The listing builds one solid part. Answer for the finished solid, in the listing's coordinates (mm). Give positions to 0.01 mm unless a question says otherwise; leave off trailing zeros. Write each loop counter-clockwise with the first axis right and the second up, starting at its lowest first coordinate (ties: lowest second). Pieces come first, ordered by that corner, then holes. Notation, with made-up numbers: (-31, 60) -> (2, 60) arc R9 cw to (2, 71) -> close; hole circle Ø5 at (81.5, 73). An arc over 180 degrees is marked (long way). One line per question, with ' | ' between items.
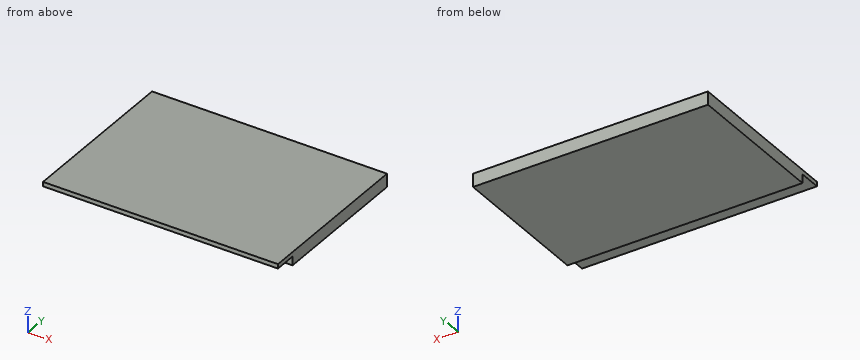
from build123d import *

# Parameters (mm, degrees)
F0_W     = 127
F0_H     = 79.375
F1_DEPTH = 7.5
F0_W_2   = 3.175
F0_H_2   = 12.7
F2_DEPTH = 2.5


with BuildPart() as f1:
    # F0 (on Top) → F1 (new body)
    with BuildSketch(Plane.XY):
        Polygon((85.0653162807, 76.807467067), (-48.2846837193, 76.807467067), (-48.2846837193, -5.742532933), (-45.1096837193, -5.742532933), (-45.1096837193, 73.632467067), (81.8903162807, 73.632467067), (81.8903162807, -5.742532933), (85.0653162807, -5.742532933), align=None)
        with Locations((18.3903162807, 33.944967067)):
            Rectangle(F0_W, F0_H)
    extrude(amount=-F1_DEPTH)

    # F0 (on Top) → F2 (join)
    with BuildSketch(Plane.XY):
        with Locations((-46.6971837193, -12.092532933)):
            Rectangle(F0_W_2, F0_H_2)
        with Locations((83.4778162807, -12.092532933)):
            Rectangle(F0_W_2, F0_H_2)
        with Locations((18.3903162807, -12.092532933)):
            Rectangle(F0_W, F0_H_2)
    extrude(amount=-F2_DEPTH)


solid = f1.part
Item 1: A flat-ended cylindrical pin translates along its axis: pin 1 (6 mm diameter, centred on x = 32, y = 15.5, fed in from +Z). Find the tip coordinate at first contact, or state that the pin passes through.
Answers below:
pin 1: z = 0
Item 2: Find section B-B (z = -6.25). Write down the section's boundary in (x, y), then the cut area to 3 significant figures.
Answers below:
outline: (-48.28, -5.74) -> (85.07, -5.74) -> (85.07, 76.81) -> (-48.28, 76.81) -> close | area: 11,000 mm²
Item 3: Consider line 1 (Y direction, x = 5.5, z = -6.25); line 2 (Z direction, x = -34, y = -9). Determine where each line is inside the solid, lowest interval first. Write a range as [from, to].
Answers below:
line 1: [-5.74, 76.81] | line 2: [-2.5, 0]
Item 4: Find section A-A (x = 47.5). Write down the section's boundary in (y, z), then the cut area to 3 significant figures.
Answers below:
outline: (-18.44, -2.5) -> (-5.74, -2.5) -> (-5.74, -7.5) -> (76.81, -7.5) -> (76.81, 0) -> (-18.44, 0) -> close | area: 651 mm²
